Geometry: final body of the model. Coordinates: model frame, mm. Face numbers are marked on the shaded views. A direction names the side the tool comes from. Give positions to 0.01 mm unless a question says otherwise; leave off trailing zeros. Loops run counter-clockwise (first coordinate to the right, second up) from the corner with the lowest first, then second, coordinate; pieces in that order, holes last. Notation, with made-up numbers: (1.25, 78.25) -> (51.25, 78.25) arc R29 ccw to (51.25, 112.25) -> close; hole circle Ø9 at (2.25, 75.25). An arc over 180 degrees is marked (long way). Answer in a Markdown table with one row per item. Add a question column.
1) First-contact query: P1, Ø3, axis at x = 22.5, z = 72.5, coming from the +Y side; P2, Ø0.6, axis at x = 0, y = 18.5, coming from the -Z side; P3, Ø1, axis at x = -1.5, z = 53, coming from the -Y side. Flat tips, straight axial feed; report the tip coordinate or a pass-through.
2) Section query B-B (y = 2). Return the cut outline in (x, z).
3) Draft query along X for the marked faces 3, 4 and 5. Return one class per face: +X half, -X half, draft (parallel to the pull), parting line (faces both ways), or undercut.
4) Access query for the marked faces 1 and 2. Directions: +Z, -Z, +X, -X, +Y, -Y. A direction counts if a zero-diameter tool reaches every point of the face in a straight line with its end or side. Return the directions, or none.
5) Line query: line 1 (Y direction, x = 15, z = 17); line 2 (X direction, y = 8.5, z = 54.5); line 3 (Y direction, x = -4.5, z = 95). Output: solid intervals per line, ascending. Write a range as from..to.
6) Section query C-C (y = -13). Return the cut outline in (x, z).
7) Section query A-A (z = 12). Return the cut outline in (x, y).
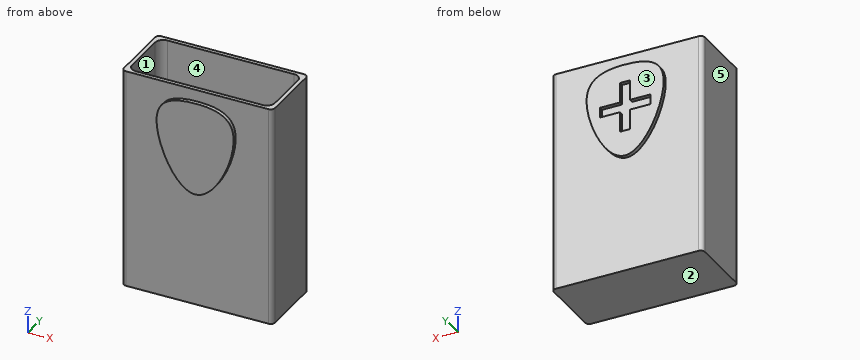
```python
from build123d import *

# Parameters (mm, degrees)
F0_W      = 75
F0_H      = 34
F2_DEPTH  = 110
F3_W      = 71
F3_H      = 30
F4_DEPTH  = 108
F5_R      = 2
F6_R      = 4
F8_DEPTH  = 2
F10_W     = 5
F10_H     = 10
F10_W_2   = 10
F10_H_2   = 5
F11_DEPTH = 2


with BuildPart() as f2:
    # F0 (on Top) → F2 (new body)
    with BuildSketch(Plane.XY):
        Rectangle(F0_W, F0_H)
    extrude(amount=F2_DEPTH)

    # F3 (on face) → F4 (cut)
    with BuildSketch(Plane.XY.offset(110)):
        Rectangle(F3_W, F3_H)
    extrude(amount=-F4_DEPTH, mode=Mode.SUBTRACT)

    # F5
    f5_edges = [f2.edges().sort_by_distance(p)[0] for p in [
        (-37.5, 17, 55),
        (37.5, 17, 55),
        (37.5, -17, 55),
        (-37.5, -17, 55),
    ]]
    fillet(f5_edges, radius=F5_R)

    # F6
    f6_edges = [f2.edges().sort_by_distance(p)[0] for p in [
        (-35.5, 15, 56),
        (-35.5, -15, 56),
        (35.5, 15, 56),
        (35.5, -15, 56),
    ]]
    fillet(f6_edges, radius=F6_R)

    # F7 (on face) → F8 (join)
    with BuildSketch(Plane.XZ.offset(17)):
        with BuildLine():
            add(Edge.make_bspline(
                [(18.7785252929, 94.3015664816), (17.0131724762, 102.694836153), (0, 105.7685942517), (-28.8612375736, 100.5542544303), (0, 32.6291322034), (21.2373277439, 82.6113299209), (18.7785252929, 94.3015664816)],
                knots=[0, 0, 0, 0, 0.2089592717, 0.4179185434, 0.7089592717, 1, 1, 1, 1], degree=3))
        make_face()
    extrude(amount=F8_DEPTH)

    # F9: F2 across plane


with BuildPart() as f2_1:
    add(f2.part)
    add(f2.part.mirror(Plane.XZ))

    # F10 (on face) → F11 (cut)
    with BuildSketch(Plane(origin=(0, 19, 0), x_dir=(-1, 0, 0), z_dir=(0, 1, 0))):
        with Locations((0, 90.4341701968)):
            Rectangle(F10_W, F10_H)
        with Locations((-7.5, 82.9341701968)):
            Rectangle(F10_W_2, F10_H_2)
        with Locations((0, 82.9341701968)):
            Rectangle(F10_W, F10_H_2)
        with Locations((7.5, 82.9341701968)):
            Rectangle(F10_W_2, F10_H_2)
        with Locations((0, 75.4341701968)):
            Rectangle(F10_W, F10_H)
    extrude(amount=-F11_DEPTH, mode=Mode.SUBTRACT)


solid = f2_1.part
```
Evaluation:
| question | item | result |
|---|---|---|
| 1 | P1 | y = 17 |
| 1 | P2 | z = 57.62 |
| 1 | P3 | y = -17 |
| 2 | outline | (-37.5, 0) -> (37.5, 0) -> (37.5, 110) -> (35.5, 110) -> (35.5, 2) -> (-35.5, 2) -> (-35.5, 110) -> (-37.5, 110) -> close |
| 3 | face 3 | draft |
| 3 | face 4 | undercut |
| 3 | face 5 | -X half |
| 4 | face 1 | +Z |
| 4 | face 2 | -Z, +X, -X, +Y, -Y |
| 5 | line 1 | -17..-15, 15..17 |
| 5 | line 2 | -37.5..-35.5, 35.5..37.5 |
| 5 | line 3 | -19..-15, 15..19 |
| 6 | outline | (-37.5, 0) -> (37.5, 0) -> (37.5, 110) -> (34.96, 110) -> (34.96, 2) -> (-34.96, 2) -> (-34.96, 110) -> (-37.5, 110) -> close |
| 7 | outline | (-37.5, -15) arc R2 ccw to (-35.5, -17) -> (35.5, -17) arc R2 ccw to (37.5, -15) -> (37.5, 15) arc R2 ccw to (35.5, 17) -> (-35.5, 17) arc R2 ccw to (-37.5, 15) -> close; hole (-35.5, -11) arc R4 ccw to (-31.5, -15) -> (31.5, -15) arc R4 ccw to (35.5, -11) -> (35.5, 11) arc R4 ccw to (31.5, 15) -> (-31.5, 15) arc R4 ccw to (-35.5, 11) -> close |
